Job drawing, mm, ordinate dimensions from the low corner. One solid piece. A direction names the side the tool comes from. Coordinates: 2 decimals unless noted, no trailing zeros. Order: outer loops, then holes, each group sorted by start corner. A loop starts at its lowest first (then second) coordinate and runs counter-clockwise, first axis right, second up. Notation, with made-up numbers: (1, 5.25) - (50, 5.25) arc R22 cw to (50, 13.25) - close; hole circle Ø5 at (59.25, -20.5). An arc over 180 degrees is marked (long way). Use one line per item in the form item = value.
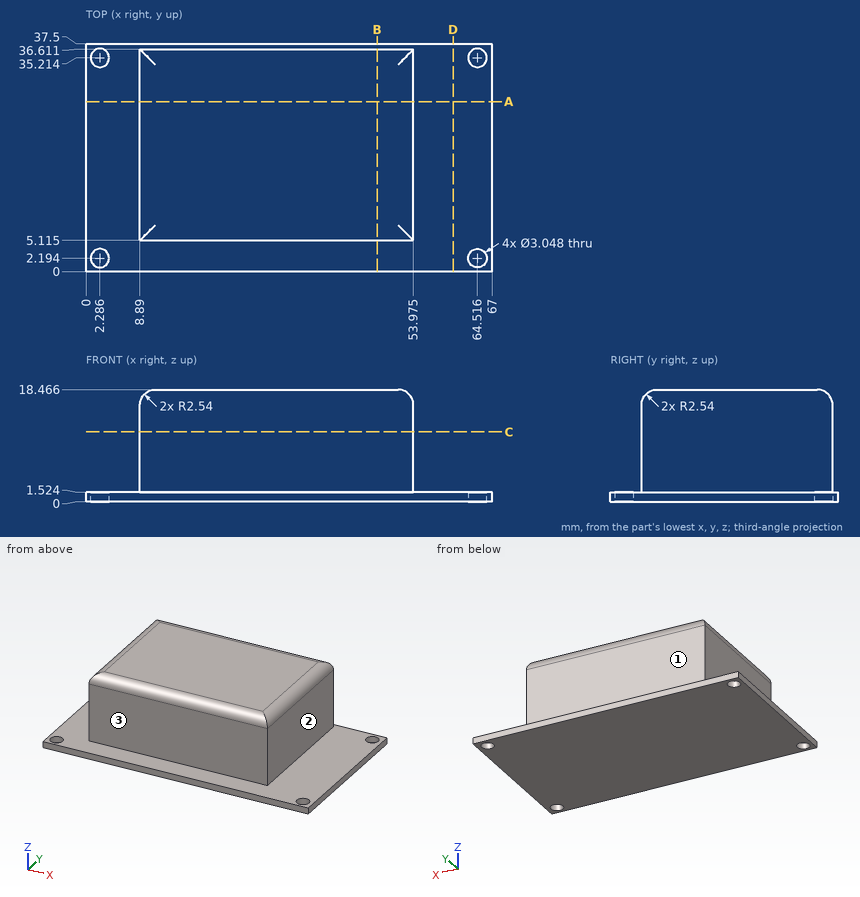
Item 1: Drop flat-ended pins along their axis: pin 1 (1 mm diameter, centred on y = 31.5, z = 12, fed in from +X) (3 decimals); pin 2 (4 mm diameter, centred on x = 2.286, y = 2.194, fed in from +Z); pin 3 (4 mm diameter, centred on x = 43, z = 13, fed in from +Y); pin 4 (8 mm diameter, centred on y = 33, z = 4.5, fed in from -X). Give the stop position or say it passes through.
Derived:
pin_1 = 53.975
pin_2 = 1.52
pin_3 = 36.61
pin_4 = 0
Item 2: 3-axis set-ups, long thin cutter, end or side, ignore diameter. For the marked faces 1, 2 and 3: which of +Z, -Z, +X, -X, +Y, -Y reach the whole face in a straight line?
Derived:
face_1 = +Z, +X, -X, +Y
face_2 = +Z, +X, +Y, -Y
face_3 = +Z, +X, -X, -Y
Item 3: Drill centre lines: line 1 (Y direction, x = 36, z = 9) (3 decimals); line 2 (Z direction, x = 11, y = 3); line 3 (X direction, y = 23.5, z = 11.5) (3 decimals). Where is each one in solid material? Low to high. Write a range as [from, to].
Derived:
line_1 = [5.115, 36.611]
line_2 = [0, 1.52]
line_3 = [8.89, 53.975]
Item 4: Cut at B-B, the plane x = 48. Write the cut outline in (y, z) (1 decimal).
Derived:
outline = (0, 0) - (37.5, 0) - (37.5, 1.5) - (36.6, 1.5) - (36.6, 15.9) arc R2.5 ccw to (34.1, 18.5) - (7.7, 18.5) arc R2.5 ccw to (5.1, 15.9) - (5.1, 1.5) - (0, 1.5) - close
Item 5: Cut at D-D, the plane x = 60.5. Write the cut outline in (y, z).
Derived:
outline = (0, 0) - (37.5, 0) - (37.5, 1.52) - (0, 1.52) - close
Item 6: Cut at A-A, the plane y = 28. Write the cut outline in (x, z) (1 decimal).
Derived:
outline = (0, 0) - (67, 0) - (67, 1.5) - (54, 1.5) - (54, 15.9) arc R2.5 ccw to (51.4, 18.5) - (11.4, 18.5) arc R2.5 ccw to (8.9, 15.9) - (8.9, 1.5) - (0, 1.5) - close
Item 7: Cut at C-C, the plane z = 11.5. Write the cut outline in (x, y) (3 decimals).
Derived:
outline = (8.89, 5.115) - (53.975, 5.115) - (53.975, 36.611) - (8.89, 36.611) - close
